```python
from build123d import *

# Parameters (mm, degrees)
SKETCH_1_R          = 12
EXTRUDE_1_DEPTH     = 25
CUT_EXTRUDE_START   = -5
CUT_EXTRUDE_1_DEPTH = 5
SKETCH_4_W          = 52.563829399
SKETCH_4_H          = 76.236989851
SKETCH_4_W_2        = 57.767152805
SKETCH_4_H_2        = 93.721065463
CUT_EXTRUDE_5_DEPTH = 5
SKETCH_5_W          = 450
SKETCH_5_H          = 40
CUT_EXTRUDE_6_DEPTH = 10
SKETCH_7_W          = 450
SKETCH_7_H          = 40
CUT_EXTRUDE_7_DEPTH = 10


with BuildPart() as part:
    # 草图1 → 凸台-拉伸1 (new body)
    with BuildSketch(Plane.XY):
        with BuildLine():
            Line((20.000001136, 44.999994952), (-4.390239864, 39.512196031))
            ThreePointArc((-4.390239864, 39.512196031), (-20, 20), (-4.390239864, 0.487803969))
            Line((-4.390239864, 0.487803969), (20.000001136, -4.999994952))
            Line((20.000001136, -4.999994952), (479.999998864, -4.999994952))
            Line((479.999998864, -4.999994952), (504.390239864, 0.487803969))
            ThreePointArc((504.390239864, 0.487803969), (520, 20), (504.390239864, 39.512196031))
            Line((504.390239864, 39.512196031), (479.999998864, 44.999994952))
            Line((479.999998864, 44.999994952), (20.000001136, 44.999994952))
        make_face()
        with Locations((0, 20)):
            Circle(SKETCH_1_R, mode=Mode.SUBTRACT)
        with Locations(Location((500, 20, 0), (0, 0, 180))):
            Circle(SKETCH_1_R, mode=Mode.SUBTRACT)
    extrude(amount=EXTRUDE_1_DEPTH)

    # 草图2 → 切除-拉伸1 (cut)
    with BuildSketch(Plane.XY.offset(25).offset(CUT_EXTRUDE_START)):
        with BuildLine():
            Line((-4.390239864, 39.512196031), (20.000001136, 44.999994952))
            Line((20.000001136, 44.999994952), (20.000001136, -4.999994952))
            Line((20.000001136, -4.999994952), (-4.390239864, 0.487803969))
            ThreePointArc((-4.390239864, 0.487803969), (-20, 20), (-4.390239864, 39.512196031))
        make_face()
        with BuildLine():
            Line((504.390239864, 39.512196031), (479.999998864, 44.999994952))
            Line((479.999998864, 44.999994952), (479.999998864, -4.999994952))
            Line((479.999998864, -4.999994952), (504.390239864, 0.487803969))
            ThreePointArc((504.390239864, 0.487803969), (520, 20), (504.390239864, 39.512196031))
        make_face()
    extrude(amount=CUT_EXTRUDE_1_DEPTH, mode=Mode.SUBTRACT)

    # 草图4 → 切除-拉伸5 (cut)
    with BuildSketch(Plane(origin=(0, 0, 0), x_dir=(-1, 0, 0), z_dir=(0, 0, -1))):
        with Locations((-506.281913563, 33.118499974)):
            Rectangle(SKETCH_4_W, SKETCH_4_H)
        with Locations((8.883575266, 41.86053778)):
            Rectangle(SKETCH_4_W_2, SKETCH_4_H_2)
    extrude(amount=-CUT_EXTRUDE_5_DEPTH, mode=Mode.SUBTRACT)

    # 草图5 → 切除-拉伸6 (cut)
    with BuildSketch(Plane(origin=(0, 0, 0), x_dir=(-1, 0, 0), z_dir=(0, 0, -1))):
        with Locations((-250.000001136, 19.999994952)):
            Rectangle(SKETCH_5_W, SKETCH_5_H)
    extrude(amount=-CUT_EXTRUDE_6_DEPTH, mode=Mode.SUBTRACT)

    # 草图7 → 切除-拉伸7 (cut)
    with BuildSketch(Plane.XY.offset(25)):
        with Locations((250.000001136, 20.000005048)):
            Rectangle(SKETCH_7_W, SKETCH_7_H)
    extrude(amount=-CUT_EXTRUDE_7_DEPTH, mode=Mode.SUBTRACT)


solid = part.part
```
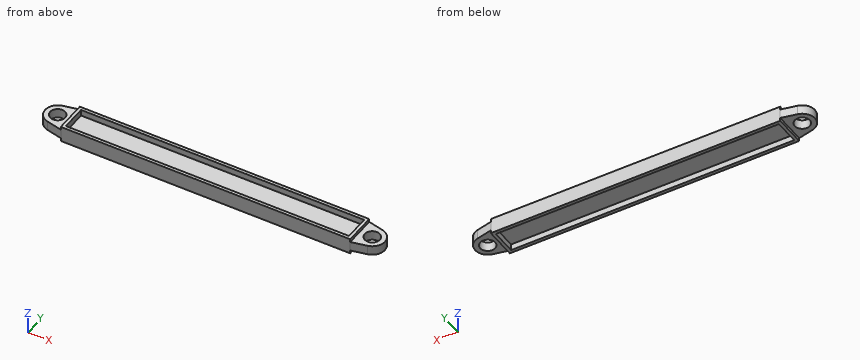
CAD build for the part. Positions are in the model's coordinates, mm. Coordinates: 2 decimals unless noted, no trailing zeros. Order: outer loops, then holes, each group sorted by start corner. A loop starts at its lowest first (then second) coordinate and runs counter-clockwise, first axis right, second up. Notation, with made-up numbers: (19, 34) -> (74, 34) arc R17 cw to (74, 54) -> close; hole circle Ø1 at (24.5, 79.5). An arc over 180 degrees is marked (long way). Use one line per item in the form item = value. Start each with the question number.
1) Drill centre lines: L1, parallel to Y at x = 423, z = 6; L2, parallel to X at y = 28, z = 16.5; L3, parallel to X at y = 22, z = 8.5. Where is each one in solid material? Low to high. Write a range as [from, to].
2) Band-saw the part on A-A on x = 500. Give the cut face in (y, z).
3) Band-saw the part on B-B on y = 20. Give the cut face in (x, z).
4) Drop flat-ended pins along their axis: pin 1 (2.5 mm diameter, centred on y = 11.5, z = 2.5, fed in from +X); pin 2 (8 mm diameter, centred on y = 14, z = 22, fed in from +X); pin 3 (2.5 mm diameter, centred on y = 28, z = 3.5, fed in from -X); pin 4 (14.5 mm diameter, centred on x = 0, y = 20, fed in from -Z). Give the stop position or say it passes through.
5) Band-saw the part on C-C on x = 166. Give the cut face in (y, z).
Entries:
q1.L1 = [-5, 0], [40, 45]
q1.L2 = [-18.33, -8.94], [8.94, 25], [475, 491.06], [508.94, 518.33]
q1.L3 = [-19.9, -11.83], [11.83, 25], [475, 488.17], [511.83, 519.9]
q2.outline = (-0.5, 5) -> (8, 5) -> (8, 20) -> (-0.5, 20) -> close; (32, 5) -> (40.5, 5) -> (40.5, 20) -> (32, 20) -> close
q3.outline = (-20, 5) -> (-12, 5) -> (-12, 20) -> (-20, 20) -> close; (12, 5) -> (20, 5) -> (20, 0) -> (25, 0) -> (25, 10) -> (475, 10) -> (475, 0) -> (480, 0) -> (480, 5) -> (488, 5) -> (488, 20) -> (480, 20) -> (480, 25) -> (475, 25) -> (475, 15) -> (25, 15) -> (25, 25) -> (20, 25) -> (20, 20) -> (12, 20) -> close; (512, 5) -> (520, 5) -> (520, 20) -> (512, 20) -> close
q4.pin_1 = 480
q4.pin_2 = 519.84
q4.pin_3 = 20
q4.pin_4 = through
q5.outline = (-5, 0) -> (0, 0) -> (0, 10) -> (40, 10) -> (40, 0) -> (45, 0) -> (45, 25) -> (40, 25) -> (40, 15) -> (0, 15) -> (0, 25) -> (-5, 25) -> close
